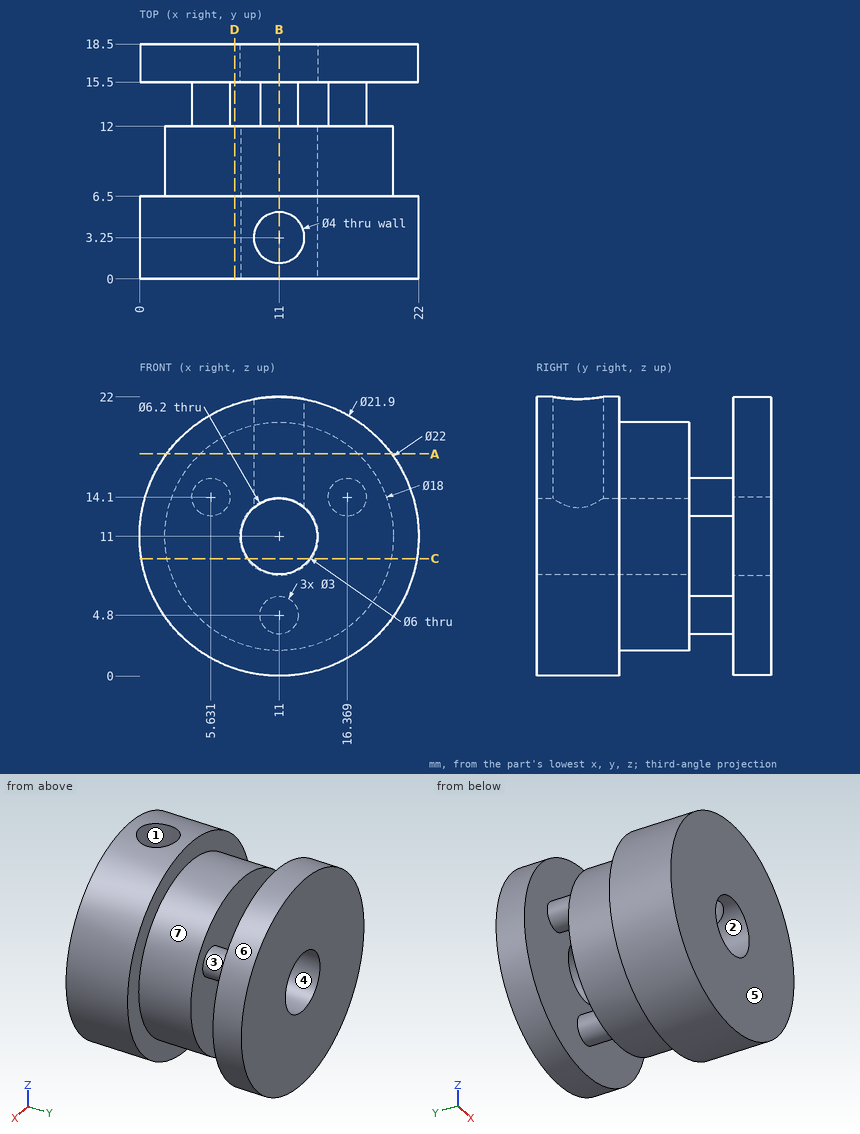
Geometry check sheet. Reference: drawing and pictorial views, mm from the part's lowest x, y, z. A direction names the side the tool comes from. Round coordinates to 2 decimals unless told otherwise and drop trailing zeros. Loops run counter-clockwise (first coordinate to the right, second up) from the corner with the lowest first, then second, coordinate; pieces in that order, holes last. Notation, with made-up numbers: (27, 75) -> (85, 75) arc R24 cw to (85, 91) -> close; hole circle Ø5 at (70, 14.5). An arc over 180 degrees is marked (long way). Answer as a JSON object with one key per item and string values. Group by question number.
Item 1: Thickness scan on line 1 along Y through (x, z) = (11, 19); line 2 along Y through (x, z) = (14.75, 9); line 3 along Z through (x, y) = (11, 17). Record the ranges inside material, lowest first.
Item 2: Cross-section at A-A, the plane z = 17.5. Count the separate pieces of the cut face and the enclosed holes in it, plus the area to 3 significant figures.
Item 3: Cross-section at D-D, the plane x = 7.5. Record the cut outline in (y, z) (1 decimal), plus the area to 3 significant figures.
Item 4: Cross-section at C-C, the plane z = 9.25. Record the cut outline in (x, y), plus the area to 3 significant figures.
Item 5: Release check for a two-part mould opening along Y. For the marked faces 5, 6 and 7 record: pulls with the +Y half, pulls with the -Y half, needs draft (parallel to the pull), parting line crosses it, or undercut.
Item 6: Set-up check for the marked faces 1, 2, 3 and 4: record each of +Z, -Z, +X, -X, +Y, -Y from which the full face is reachable in a straight line by a thin tool's end or side.
Item 7: Depth check by flat-ended pin: pin 1 Ø3 at (x, y) = (11, 3.25) entering from +Z; pin 2 Ø5.5 at (x, z) = (11, 11) entering from -Y; pin 3 Ø5 at (x, y) = (3, 9.5) entering from -Z (1 decimal); pin 4 Ø8 at (y, z) = (16.5, 6) entering from -X. Enter the tip coordinate at first touch or a pass-through.
Item 8: Cross-section at B-B, the plane x = 11. Record the cut outline in (y, z).
Determined:
{
 "1": {"line 1": "y = 0 to 1.25, 5.25 to 12, 15.5 to 18.5", "line 2": "y = 0 to 12, 15.5 to 18.5", "line 3": "z = 0.05 to 7.9, 14.1 to 21.95"},
 "2": {"separate pieces": "2", "enclosed holes": "1", "area": "224 mm²"},
 "3": {"outline": "(0, 0.6) -> (6.5, 0.6) -> (6.5, 2.7) -> (12, 2.7) -> (12, 19.3) -> (6.5, 19.3) -> (6.5, 21.4) -> (0, 21.4) -> close; (15.5, 0.6) -> (18.5, 0.6) -> (18.5, 21.4) -> (15.5, 21.4) -> close", "area": "289 mm²"},
 "4": {"outline": "(0.14, 0) -> (8.56, 0) -> (8.56, 12) -> (2.17, 12) -> (2.17, 6.5) -> (0.14, 6.5) -> close; (0.19, 15.5) -> (8.44, 15.5) -> (8.44, 18.5) -> (0.19, 18.5) -> close; (13.44, 0) -> (21.86, 0) -> (21.86, 6.5) -> (19.83, 6.5) -> (19.83, 12) -> (13.44, 12) -> close; (13.56, 15.5) -> (21.81, 15.5) -> (21.81, 18.5) -> (13.56, 18.5) -> close", "area": "229 mm²"},
 "5": {"face 5": "pulls with the -Y half", "face 6": "needs draft", "face 7": "undercut"},
 "6": {"face 1": "+Z", "face 2": "+Y, -Y", "face 3": "none", "face 4": "+Y"},
 "7": {"pin 1": "stops at z = 8.4", "pin 2": "passes through", "pin 3": "stops at z = 3.9", "pin 4": "stops at x = 0.1"},
 "8": {"outline": "(0, 0) -> (6.5, 0) -> (6.5, 2) -> (12, 2) -> (12, 3.3) -> (15.5, 3.3) -> (15.5, 0.05) -> (18.5, 0.05) -> (18.5, 7.9) -> (15.5, 7.9) -> (15.5, 6.3) -> (12, 6.3) -> (12, 8) -> (0, 8) -> close; (0, 14) -> (1.25, 14) -> (1.25, 22) -> (0, 22) -> close; (5.25, 14) -> (12, 14) -> (12, 20) -> (6.5, 20) -> (6.5, 22) -> (5.25, 22) -> close; (15.5, 14.1) -> (18.5, 14.1) -> (18.5, 21.95) -> (15.5, 21.95) -> close"}
}
